For this review, take the finished solid that the model builds, in its own axes (mm). A direction names the side the tool comes from. Give positions to 0.01 mm unless a question says otherwise; leave off trailing zeros. Order: outer loops, then holes, each group sorted by start corner. A loop starts at its lowest first (then second) coordinate and runs counter-clockwise, first axis right, second up. Notation, with made-up numbers: (87, -2) -> (121, -2) arc R25 cw to (121, 15) -> close; hole circle Ø10 at (35.5, 48.25). An arc over 180 degrees is marked (long way). Use CSV: the item, a comma, the result in double quotes. Start each with the question number.
Autodesk Inventor part; units mm, degrees
ref_plane "YZ Plane" through (0, 0, 0) normal (1, 0, 0) x (0, 1, 0)
ref_plane "XZ Plane" through (0, 0, 0) normal (0, 1, 0) x (-1, 0, 0)
ref_plane "XY Plane" through (0, 0, 0) normal (0, 0, 1) x (1, 0, 0)
sketch "Sketch_1" plane through (0, 0, 0) normal (0, 0, 1) x (1, 0, 0)
  line L0 (7, 0) -> (0, 0)
  line L1 (0, 3.3) -> (0.3, 3)
  line L2 (0.3, 3) -> (6.7, 3)
  line L3 (6.7, 3) -> (7, 3.3)
  line L4 (7, 3.3) -> (7, 3.7)
  line L5 (7, 3.7) -> (6, 4)
  line L6 (6, 4) -> (1, 4)
  line L7 (1, 4) -> (1, 6)
  line L8 (1, 6) -> (0, 6)
  line L9 (0, 6) -> (0, 3.3)
revolve "Revolution1" add sketch "Sketch_1" angle 360 about axis through (7, 0, 0) along (1, 0, 0)
sketch "스케치2" plane through (0, 0, 0) normal (-1, 0, 0) x (0, 0, 1)
  circle A0 centre (0, 0) radius 3.3
  circle A1 centre (0, 0) radius 6
  circle A2 centre (0, 0) radius 3.025
  dimension "d1" = 6.05
extrude "돌출1" cut sketch "스케치2" against normal up to surface (7 mm away) contours A2
move faces "이동1" translate (-2, 0, 0) faces at (0, 5.0099, -0.7419) (0.0917, 3.1979, -0.2582) (1, 5.2365, -0.7977) (0.6667, 5.9223, -0.9625)
move faces "이동2" translate (2, 0, 0) faces at (6.1667, -1.7292, 3.5514) (6.9083, 3.1979, -0.2582) (7, 3.5308, -0.2952)
properties part number "80F-0610"
1. Consider section C-C (x = 5.5). State the section outline as (y, z) points (3 decimals), plus the area to 3 significant figures.
2. To check wall thickness, follow L1, parallel to Z at x = 3.25, y = 0 (3 decimals); L2, parallel to X at y = -5, z = -0.5; L3, parallel to Y at x = 7.75, z = 2.75. State the ranges of each line that lie inside material, in increasing order. Write a range as [from, to].
3. Draft analysis for pull direction Y (two halves, no side actions). For faces 3 (the face through (-2, 3, -3)), 4 (the face through (3.427, 0.909, 2.885)), 5 (the face through (3.437, -0.867, 3.905)), state which applies: +Y half, -Y half, draft (parallel to the pull), parting line (faces both ways), or undercut.
4. Clearance check with flat-ended pins moving along their axes: P1, Ø3, axis at x = 7.5, y = -0.5, coming from the -Z side; P2, Ø1, axis at x = 1.5, y = 3.5, coming from the -Z side; P3, Ø1, axis at x = 4.5, y = -2, coming from the +Z side. State where each tip first meets the part, or that it passes through.
5. For faces 1 (the face through (-1.493, -5.994, 0.264)), 2 (the face through (-1, -1.42, -3.92)), list the 3-axis set-ups (+Z, -Z, +X, -X, +Y, -Y) from which the entire face can be reached by the end or side of a thin tool; tool diameter is ignored.
6. Consider section D-D (y = -4.5). State the section outline as (x, z) points, plus the area to 3 significant figures.
7. Consider section A-A (z = 0). State the section outline as (x, y) points (3 decimals), plus the area to 3 significant figures.
Answer list:
1,outline,"circle Ø8 at (0, 0); hole circle Ø6.05 at (0, 0)"
1,area,"21.5 mm2"
2,L1,"[-4, -3.025], [3.025, 4]"
2,L2,"[-2, -1]"
2,L3,"[-2.9, -1.26], [1.26, 2.9]"
3,face 3,"draft"
3,face 4,"undercut"
3,face 5,"parting line"
4,P1,"z = -4"
4,P2,"z = -2.65"
4,P3,"z = 3.71"
5,face 1,"+X, -X"
5,face 2,"+X"
6,outline,"(-2, -3.97) -> (-1, -3.97) -> (-1, 3.97) -> (-2, 3.97) -> close"
6,area,"7.94 mm2"
7,outline,"(-2, -6) -> (-1, -6) -> (-1, -4) -> (8, -4) -> (9, -3.7) -> (9, -3.3) -> (8.725, -3.025) -> (-1.725, -3.025) -> (-2, -3.3) -> close; (-2, 3.3) -> (-1.725, 3.025) -> (8.725, 3.025) -> (9, 3.3) -> (9, 3.7) -> (8, 4) -> (-1, 4) -> (-1, 6) -> (-2, 6) -> close"
7,area,"25.0 mm2"
